Build history of the part. All positions in model axes, mm. A direction names the side the tool comes from. Give positions to 0.01 mm unless a question says otherwise; leave off trailing zeros. Loops run counter-clockwise (first coordinate to the right, second up) from the corner with the lowest first, then second, coordinate; pieces in that order, holes last. Notation, with made-up numbers: (9.5, -35.75) -> (18.5, -35.75) arc R27 ccw to (18.5, -11.75) -> close; hole circle Ø7 at (8.5, -12.5). An arc over 180 degrees is marked (long way). Answer as a JSON object with one key per item and string values. Group by question number.
Q1. Drop flat-ended pins along their axis: pin 1 (6 mm diameter, centred on x = 2, z = 6.5, fed in from -Y); pin 2 (11.5 mm diameter, centred on x = 0, y = 57, fed in from +Z); pin 3 (6 mm diameter, centred on x = -8, z = 6.5, fed in from +Y); pin 4 (2 mm diameter, centred on y = 48.5, z = 9, fed in from +X). Give the stop position or say it passes through.
Q2. Tool access for faces 1 (the cylindrical face through (1.301, 51.143, 3.549)), 2 (the flat face through (-4.2, 61.5, 7)): list every direction of +Z, -Z, +X, -X, +Y, -Y with a clear straight run to the whole face (end or side of a thin tool).
Q3. Wall check: probe 1 along Y at (x, z) = (0, 1.5); probe 2 along Y at (x, z) = (0, 8.25); probe 3 along X at (y, z) = (51.5, 1.25). Give the ranges that are in metal, low to high. Write a range as from..to.
Q4. Band-saw the part on B-B, the plane y = 57. Write the cut outline in (x, z), plus the area to 4 significant figures.
Q5. Band-saw the part on C-C, the plane z = 5. Write the cut outline in (x, y).
Q6. Band-saw the part on D-D, the plane y = 50. Write the cut outline in (x, z).
Q7. Band-saw the part on A-A, the plane x = 0. Write the cut outline in (y, z), plus the area to 4 significant figures.
Q8. Two-plate mould, pull along X, no slides. Class faces 3 (the cylindrical face through (-5.24, 65.22, 8.52)), 4 (the flat face through (-4.5, 47.7, 10)), 5 (the cylindrical face through (2.799, 78.317, 5.07)): pulls with the +X half, pulls with the -X half, needs draft (parallel to the pull), parting line crosses it, or undercut.
from build123d import *

# Parameters (mm, degrees)
CYLINDER005_R          = 6
CYLINDER005_DEPTH      = 20
CYLINDER007_R          = 9.75
CYLINDER007_DEPTH      = 6
CYLINDER003_R          = 21.5
CYLINDER003_DEPTH      = 10
CUT003_PLACEMENT_ANGLE = 180


with BuildPart() as cylinder005:
    # Cylinder005 → Cylinder005 (new body)
    with BuildSketch(Plane.XY):
        Circle(CYLINDER005_R)
    extrude(amount=CYLINDER005_DEPTH)


with BuildPart() as cylinder007:
    # Cylinder007 → Cylinder007 (new body)
    with BuildSketch(Plane.XY):
        Circle(CYLINDER007_R)
    extrude(amount=CYLINDER007_DEPTH)


with BuildPart() as large_bearing_ring:
    # Cylinder003 → Cylinder003 (new body)
    with BuildSketch(Plane.XY.offset(3)):
        Circle(CYLINDER003_R)
    extrude(amount=CYLINDER003_DEPTH)

    # Cut002: cut Cylinder007
    add(cylinder007.part, mode=Mode.SUBTRACT)

    # Cut003: cut Cylinder005
    add(cylinder005.part, mode=Mode.SUBTRACT)


with BuildPart() as large_bearing_ring_1:
    # Cut003 placement: moved
    add(large_bearing_ring.part.moved(Location((0, 57, 13))).rotate(Axis((0, 57, 13), (0, 1, 0)), CUT003_PLACEMENT_ANGLE))


solid = large_bearing_ring_1.part
Worked answers:
{
 "1": {"pin 1": "y = 35.5", "pin 2": "through", "pin 3": "y = 77.91", "pin 4": "x = 20.15"},
 "2": {"face 1": "+Z, -Z", "face 2": "+Z"},
 "3": {"probe 1": "35.5..51, 63..78.5", "probe 2": "35.5..47.25, 66.75..78.5", "probe 3": "-20.78..-2.4, 2.4..20.78"},
 "4": {"outline": "(-21.5, 0) -> (-6, 0) -> (-6, 7) -> (-9.75, 7) -> (-9.75, 10) -> (-21.5, 10) -> close; (6, 0) -> (21.5, 0) -> (21.5, 10) -> (9.75, 10) -> (9.75, 7) -> (6, 7) -> close", "area": "287.5 mm2"},
 "5": {"outline": "circle Ø43 at (0, 57); hole circle Ø12 at (0, 57)"},
 "6": {"outline": "(-20.33, 0) -> (20.33, 0) -> (20.33, 10) -> (6.79, 10) -> (6.79, 7) -> (-6.79, 7) -> (-6.79, 10) -> (-20.33, 10) -> close"},
 "7": {"outline": "(35.5, 0) -> (51, 0) -> (51, 7) -> (47.25, 7) -> (47.25, 10) -> (35.5, 10) -> close; (63, 0) -> (78.5, 0) -> (78.5, 10) -> (66.75, 10) -> (66.75, 7) -> (63, 7) -> close", "area": "287.5 mm2"},
 "8": {"face 3": "undercut", "face 4": "needs draft", "face 5": "parting line crosses it"}
}
